The model under review builds one solid part; all positions refer to its coordinate system, in mm. Face numbers are marked on the shaded views. Round coordinates to 2 decimals unless told otherwise and drop trailing zeros. Write each loop counter-clockwise with the first axis right and the second up, starting at its lowest first coordinate (ties: lowest second). Pieces come first, ordered by that corner, then holes. Notation, with made-up numbers: (40.25, -36.75) -> (92.25, -36.75) arc R19 ccw to (92.25, -30.75) -> close; hole circle Ø8 at (28.5, 40). An arc over 180 degrees is marked (long way). Use CSV: the item, a comma, the result in double quotes. Start each with the question number.
1) Wall thickness on probe 1 along X at (y, z) = (21, 0); probe 2 along X at (y, z) = (21, -79): over which ranges is each line inside the solid? List them lowest first. Write a range as [from, to].
2) Take a section at C-C, the plane y = 16. Give the boundary of the cut face in (x, z), then the cut area to 3 significant figures.
3) Mouldability with a two-part tool opening along Z and no side actions: class the marked faces 1 and 2 as released by +Z, released by -Z, zero draft, split by the parting line, or undercut.
4) For pin 1 Ø8 at (y, z) = (24.5, 165) entering from -X; pin 2 Ø3 at (x, y) = (-73, 8.5) entering from -Z; pin 3 Ø8 at (x, z) = (28, -60.5) entering from -Y; pin 4 Ø1 at (x, y) = (-38.5, 25) entering from -Z, all flat-tipped, find the tip position at first contact; note any pin that passes through.
from build123d import *

# Parameters (mm, degrees)
SKETCH1_R           = 225
BOSS_EXTRUDE1_DEPTH = 30
SKETCH2_R           = 220
CUT_EXTRUDE1_DEPTH  = 20
SKETCH4_W           = 150
SKETCH4_H           = 10
BOSS_EXTRUDE3_DEPTH = 290
FILLET1_R           = 10
FILLET2_R           = 5


with BuildPart() as part:
    # Sketch1 → Boss-Extrude1 (new body)
    with BuildSketch(Plane(origin=(0, 0, 0), x_dir=(1, 0, 0), z_dir=(0, 1, 0))):
        with Locations(Location((0, 0, 0), (0, 0, 270))):
            Circle(SKETCH1_R)
    extrude(amount=BOSS_EXTRUDE1_DEPTH)

    # Sketch2 → Cut-Extrude1 (cut)
    with BuildSketch(Plane(origin=(0, 30, 0), x_dir=(1, 0, 0), z_dir=(0, 1, 0))):
        with Locations(Location((0, 0, 0), (0, 0, 270))):
            Circle(SKETCH2_R)
    extrude(amount=-CUT_EXTRUDE1_DEPTH, mode=Mode.SUBTRACT)

    # Sketch4 → Boss-Extrude3 (add)
    with BuildSketch(Plane.XY):
        with Locations((0, 5)):
            Rectangle(SKETCH4_W, SKETCH4_H)
    extrude(amount=BOSS_EXTRUDE3_DEPTH)

    # Fillet1
    fillet1_edges = [part.edges().sort_by_distance(p)[0] for p in [
        (75, 5, 290),
        (-75, 5, 290),
    ]]
    fillet(fillet1_edges, radius=FILLET1_R)

    # Fillet2
    fillet2_edges = [part.edges().sort_by_distance(p)[0] for p in [
        (0, 0, -225),
        (0, 30, -225),
    ]]
    fillet(fillet2_edges, radius=FILLET2_R - 0.0001)  # a hair under: the kernel refuses the full size


solid = part.part
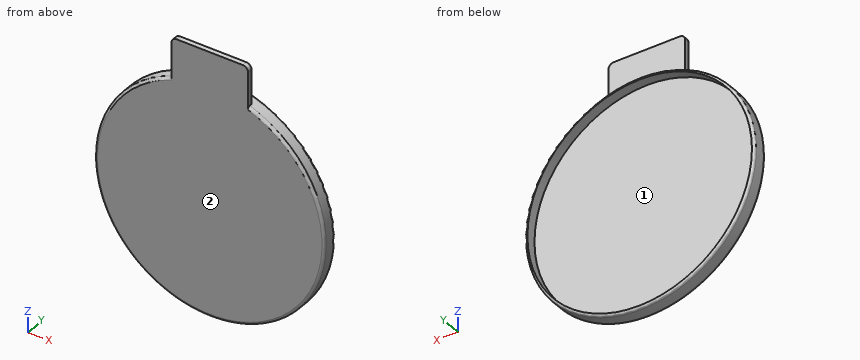
Values found:
1,probe 1,"[-225, -220], [220, 225]"
1,probe 2,"[-210.68, -205.33], [205.33, 210.68]"
2,outline,"circle Ø450 at (0, 0); hole circle Ø440 at (0, 0)"
2,area,"6,990 mm²"
3,face 1,"undercut"
3,face 2,"zero draft"
4,pin 1,"x = -157.18"
4,pin 2,"z = -213.34"
4,pin 3,"y = 0"
4,pin 4,"z = -221.77"
